```python
from build123d import *

# Parameters (mm, degrees)
BOSS_EXTRUDE1_DEPTH     = 7.5
CHAMFER1_SIZE           = 3
SKETCH2_R               = 1.8
CUT_EXTRUDE1_DEPTH      = 3
CUT_EXTRUDE1_DEPTH_BACK = 3
FILLET1_R               = 2


with BuildPart() as part:
    # Sketch1 → Boss-Extrude1 (new body, symmetric)
    with BuildSketch(Plane(origin=(0, 0, 0), x_dir=(0, 0, -1), z_dir=(1, 0, 0))):
        Polygon((-5.25, -8.75), (-5.25, -10.75), (6.75, -10.75), (6.75, 10.75), (2.25, 10.75), (2.25, 8.75), (5.25, 8.75), (5.25, 6.45), (-0.75, 6.45), (-0.75, 4.45), (5.25, 4.45), (5.25, -8.75), align=None)
    extrude(amount=BOSS_EXTRUDE1_DEPTH, both=True)

    # Chamfer1
    chamfer1_edges = [part.edges().sort_by_distance(p)[0] for p in [
        (0, -8.75, -5.25),
        (0, 4.45, -5.25),
    ]]
    chamfer(chamfer1_edges, length=CHAMFER1_SIZE)

    # Sketch2 → Cut-Extrude1 (cut, two sides)
    with BuildSketch(Plane(origin=(0, -8.75, 0), x_dir=(1, 0, 0), z_dir=(0, 1, 0))) as cut_extrude1_sk:
        with Locations((-3.7, -1.65)):
            Circle(SKETCH2_R)
        with Locations((3.7, -1.65)):
            Circle(SKETCH2_R)
    extrude(amount=CUT_EXTRUDE1_DEPTH, mode=Mode.SUBTRACT)
    extrude(cut_extrude1_sk.sketch, amount=-CUT_EXTRUDE1_DEPTH_BACK, mode=Mode.SUBTRACT)

    # Fillet1
    fillet1_edges = [part.edges().sort_by_distance(p)[0] for p in [
        (0, 10.75, -6.75),
        (0, -10.75, -6.75),
    ]]
    fillet(fillet1_edges, radius=FILLET1_R)


solid = part.part
```
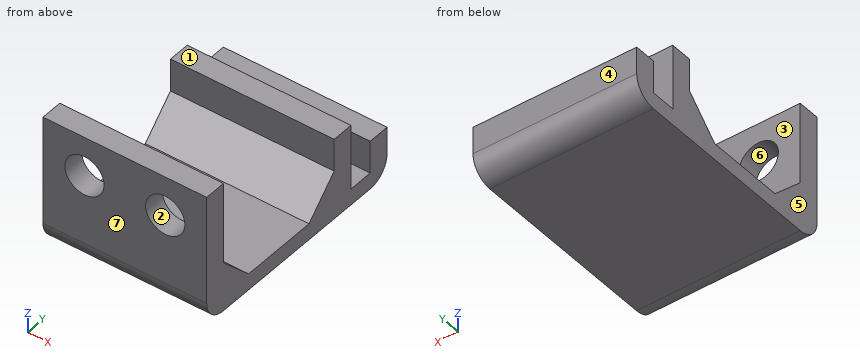
Work out the finished part from the listing and answer in its coordinate system (mm). Face numbers are marked on the shaded views. A direction names the side the tool comes from. Coordinates: 2 decimals unless noted, no trailing zeros. Write each loop counter-clockwise with the first axis right and the second up, starting at its lowest first coordinate (ties: lowest second). Pieces come first, ordered by that corner, then holes.
Q1. A cutting plane is placed at B-B, the plane x = 3.7. Give the vertices of the cut face in (y, z), then the cut area to 3 significant figures.
Q2. A cutting plane is placed at C-C, the plane z = -4. Give the vertices of the cut face in (x, y).
Q3. Find the intervals of material crossed by line 1 (X direction, y = -9.45, z = 1.65); line 2 (Y direction, x = -5.75, z = -1); line 3 (Y direction, x = 1, z = -4), in increasing order.
Q4. Determine the mould class of the marked faces 5, 6 and 7 for opening direction X: released by +X, released by -X, zero draft, split by the parting line, or undercut.
Q5. A cutting plane is placed at A-A, the plane z = -2. Give the vertices of the cut face in (x, y), then the cut area to 3 significant figures.
Q6. Which of the six approach directions +Z, -Z, +X, -X, +Y, -Y give full straight-line access (tool end or side, diameter ignored) to the marked faces 1, 2, 3 and 4?
Q7. Each of these flat-tipped pins is pushed along its axis until it touches: pin 1 Ø2 at (x, z) = (1, 2) entering from +Y; pin 2 Ø0.7 at (x, y) = (1, 8) entering from +Z; pin 3 Ø2 at (x, y) = (-2.5, 5.5) entering from +Z. Where does it stop, or does it pass through?
Q8. A cutting plane is placed at D-D, the plane x = -1.5. Give the vertices of the cut face in (y, z).
Findings below:
1. outline: (-10.75, -4.75) arc R2 ccw to (-8.75, -6.75) - (8.75, -6.75) arc R2 ccw to (10.75, -4.75) - (10.75, -2.25) - (8.75, -2.25) - (8.75, -5.25) - (6.45, -5.25) - (6.45, 0.75) - (4.45, 0.75) - (4.45, -2.25) - (1.45, -5.25) - (-5.75, -5.25) - (-8.75, -2.25) - (-8.75, -0.15) - (-10.75, -0.15) - close; (-10.75, 3.45) - (-8.75, 3.45) - (-8.75, 5.25) - (-10.75, 5.25) - close
1. area: 71.3 mm2
2. outline: (-7.5, -10.75) - (7.5, -10.75) - (7.5, -7) - (-7.5, -7) - close; (-7.5, 2.7) - (7.5, 2.7) - (7.5, 6.45) - (-7.5, 6.45) - close; (-7.5, 8.75) - (7.5, 8.75) - (7.5, 10.75) - (-7.5, 10.75) - close
3. line 1: x = -7.5 to -5.5, -1.9 to 1.9, 5.5 to 7.5
3. line 2: y = -10.75 to -8.75, 4.45 to 6.45
3. line 3: y = -10.75 to -7, 2.7 to 6.45, 8.75 to 10.75
4. face 5: released by -X
4. face 6: undercut
4. face 7: zero draft
5. outline: (-7.5, -10.75) - (7.5, -10.75) - (7.5, -8.75) - (-7.5, -8.75) - close; (-7.5, 4.45) - (7.5, 4.45) - (7.5, 6.45) - (-7.5, 6.45) - close
5. area: 60.0 mm2
6. face 1: +Z, +X, -X, +Y
6. face 2: -Y
6. face 3: +Z, +X, -X
6. face 4: +Z, -Z, +X, -X, +Y
7. pin 1: stops at y = -8.75
7. pin 2: stops at z = -5.25
7. pin 3: stops at z = 0.75
8. outline: (-10.75, -4.75) arc R2 ccw to (-8.75, -6.75) - (8.75, -6.75) arc R2 ccw to (10.75, -4.75) - (10.75, -2.25) - (8.75, -2.25) - (8.75, -5.25) - (6.45, -5.25) - (6.45, 0.75) - (4.45, 0.75) - (4.45, -2.25) - (1.45, -5.25) - (-5.75, -5.25) - (-8.75, -2.25) - (-8.75, 5.25) - (-10.75, 5.25) - close
